Check sheet for the modelled part. Datum: model origin and axes. Units: mm. Face numbers are marked on the shaded views. A direction names the side the tool comes from. Give positions to 0.01 mm unless a question says otherwise; leave off trailing zeros. Order: outer loops, then holes, each group sorted by start corner. A loop starts at its lowest first (then second) coordinate and runs counter-clockwise, first axis right, second up.
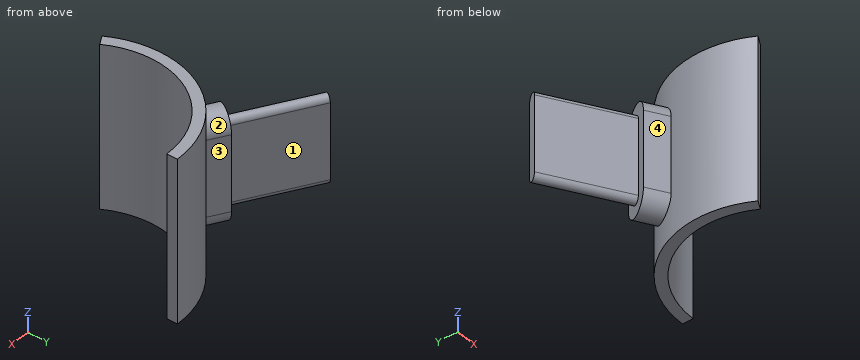
```python
from build123d import *

# Parameters (mm, degrees)
BOSS_EXTRU_1_DEPTH = 15
BOSS_EXTRU_2_START = -0.0139
BOSS_EXTRU_2_DEPTH = 10.0139
BOSS_EXTRU_4_START = -0.134477
BOSS_EXTRU_4_DEPTH = 2.134477


with BuildPart() as part:
    # Esquisse1 → Boss.-Extru.1 (new body)
    with BuildSketch(Plane.XY):
        with BuildLine():
            Line((-7.794228634, -4.5), (-6.92820323, -4))
            ThreePointArc((-6.92820323, -4), (-6.92820323, 4), (0, 8))
            Line((0, 8), (0, 9))
            ThreePointArc((0, 9), (-7.794228634, 4.5), (-7.794228634, -4.5))
        make_face()
    extrude(amount=-BOSS_EXTRU_1_DEPTH)

    # Esquisse2 → Boss.-Extru.2 (add)
    with BuildSketch(Plane(origin=(-7.794228634, 4.5, 0), x_dir=(0, 0, 1), z_dir=(-0.866025404, 0.5, 0)).offset(BOSS_EXTRU_2_START)):
        with BuildLine():
            Line((-11, 0.5), (-4, 0.5))
            ThreePointArc((-4, 0.5), (-3.5, 0), (-4, -0.5))
            Line((-4, -0.5), (-11, -0.5))
            ThreePointArc((-11, -0.5), (-11.5, 0), (-11, 0.5))
        make_face()
    extrude(amount=BOSS_EXTRU_2_DEPTH)

    # Esquisse7 → Boss.-Extru.4 (add)
    with BuildSketch(Plane(origin=(-7.794228634, 4.5, 0), x_dir=(0, 0, 1), z_dir=(-0.866025404, 0.5, 0)).offset(BOSS_EXTRU_4_START)):
        with BuildLine():
            Line((-4, 1.55), (-11, 1.55))
            ThreePointArc((-11, 1.55), (-12.55, 0), (-11, -1.55))
            Line((-11, -1.55), (-4, -1.55))
            ThreePointArc((-4, -1.55), (-2.45, 0), (-4, 1.55))
        make_face()
    extrude(amount=BOSS_EXTRU_4_DEPTH)


solid = part.part
```
(1) Cross-section at B-B on y = 2. Enter the section's corners in (x, z), then the cut area to 3 significant figures.
Response values:
outline: (-8.77, -15) - (-7.75, -15) - (-7.75, 0) - (-8.77, 0) - close
area: 15.4 mm2
(2) Cross-section at D-D on z = -11.75. Enter the section's corners in (x, y).
Response values:
outline: (-10.2, 4.33) - (-8.38, 3.27) arc R9 ccw to (-7.79, -4.5) - (-6.93, -4) arc R8 cw to (0, 8) - (0, 9) arc R9 ccw to (-7.03, 5.62) - (-8.85, 6.67) - close
(3) Cross-section at A-A on z = -6.5. Enter the section's corners in (x, y).
Response values:
outline: (-16.7, 9.07) - (-9.78, 5.07) - (-10.3, 4.16) - (-8.45, 3.09) arc R9 ccw to (-7.79, -4.5) - (-6.93, -4) arc R8 cw to (0, 8) - (0, 9) arc R9 ccw to (-6.9, 5.78) - (-8.75, 6.84) - (-9.28, 5.93) - (-16.2, 9.93) - close
(4) Cross-section at C-C on x = -1.75. Enter the section's corners in (y, z), then the cut area to 3 significant figures.
Response values:
outline: (7.81, -15) - (8.83, -15) - (8.83, 0) - (7.81, 0) - close
area: 15.3 mm2
(5) Set-up check for the marked faces 1 and 2: record each of +Z, -Z, +X, -X, +Y, -Y from which the full face is reachable in a straight line by a thin tool's end or side.
Response values:
face 1: +Z, -Z, +Y
face 2: +Z
(6) Material ranges on L1, parallel to X at y = 6.75, z = -5; L2, parallel to X at y = 6.25, z = -8; L3, parallel to X at y = 6.25, z = -3, recorded low to high.
Response values:
L1: x = -12.69 to -10.69, -8.8 to -8.59, -5.95 to -4.29
L2: x = -11.83 to -9.83, -9.09 to -7.73, -6.48 to -4.99
L3: x = -9.09 to -8.46, -6.48 to -4.99
(7) Release check for a two-part mould opening along Y. For the marked faces 3 and 4 record: released by +Y, released by -Y, zero draft, split by the parting line, or undercut.
Response values:
face 3: released by +Y
face 4: undercut
(8) Gauge pin test, flat ends, axial feed: pin 1 Ø5 at (x, z) = (-15, -10.5) entering from -Y; pin 2 Ø4 at (y, z) = (3.5, -12.5) entering from -X; pin 3 Ø3 at (x, z) = (-9, -7.5) entering from +Y; pin 4 Ø4 at (x, z) = (-6, -7.5) entering from -Y. Record the tip position at first contact, or that the pin passes through.
Response values:
pin 1: stops at y = 6.64
pin 2: stops at x = -10.3
pin 3: stops at y = 6.84
pin 4: stops at y = -4.5
